The listing builds one solid part. Answer for the finished solid, in the listing's coordinates (mm). Coordinates: 2 decimals unless noted, no trailing zeros. Order: outer loops, then holes, each group sorted by start corner. A loop starts at its lowest first (then second) coordinate and runs counter-clockwise, first axis right, second up. Notation, with made-up numbers: (33.25, -23) -> (47.25, -23) arc R33 ccw to (47.25, 12) -> close; hole circle Ø5 at (-32.75, -23). An arc over 180 degrees is marked (long way). Answer in a Markdown table with one row per item.
```python
from build123d import *

# Parameters (mm, degrees)
F0_W     = 151
F0_H     = 108
F0_R     = 6.5
F0_R_2   = 4.5
F0_R_3   = 3.5
F0_R_4   = 10.35
F0_W_2   = 22
F0_H_2   = 31
F1_DEPTH = 2


with BuildPart() as f1:
    # F0 (on Top) → F1 (new body)
    with BuildSketch(Plane.XY):
        with BuildLine():
            ThreePointArc((50.203704, -19.331837), (45.47278, -13.077209), (38.166667, -15.927249))
            ThreePointArc((38.166667, -15.927249), (41.934628, -25.586465), (50.203704, -19.331837))
        make_face()
        with BuildLine():
            ThreePointArc((50.203704, 39.331837), (41.934628, 45.586465), (38.166667, 35.927249))
            ThreePointArc((38.166667, 35.927249), (45.47278, 33.077209), (50.203704, 39.331837))
        make_face()
        Rectangle(F0_W, F0_H)
        with Locations((-43.3599, -11.497885)):
            Circle(F0_R, mode=Mode.SUBTRACT)
        with Locations((-10, -12.5)):
            Circle(F0_R_2, mode=Mode.SUBTRACT)
        with Locations((10, -27.5)):
            Circle(F0_R_2, mode=Mode.SUBTRACT)
        with BuildLine():
            ThreePointArc((32.203704, -12.260769), (21.611111, -12.941687), (24.5, -2.727922))
            ThreePointArc((24.5, -2.727922), (30.419443, -3.548953), (33.166667, -8.856181))
            ThreePointArc((33.166667, -8.856181), (32.921295, -10.625257), (32.203704, -12.260769))
        make_face(mode=Mode.SUBTRACT)
        with BuildLine():
            ThreePointArc((50.203704, -19.331837), (41.934628, -25.586465), (38.166667, -15.927249))
            ThreePointArc((38.166667, -15.927249), (45.47278, -13.077209), (50.203704, -19.331837))
        make_face(mode=Mode.SUBTRACT)
        with Locations((-50, 10)):
            Circle(F0_R_3, mode=Mode.SUBTRACT)
        with Locations((-29.722222, 0.25004)):
            Circle(F0_R, mode=Mode.SUBTRACT)
        with Locations((-29.722222, 19.74996)):
            Circle(F0_R, mode=Mode.SUBTRACT)
        with Locations((-43.3599, 31.497885)):
            Circle(F0_R, mode=Mode.SUBTRACT)
        with Locations((-62, 42)):
            Circle(F0_R_2, mode=Mode.SUBTRACT)
        with Locations((-5.846048, 33.255358)):
            Circle(F0_R_4, mode=Mode.SUBTRACT)
        with BuildLine():
            ThreePointArc((22.166667, 16.128259), (25.307228, 13.752777), (26.5, 10))
            ThreePointArc((26.5, 10), (25.307228, 6.247223), (22.166667, 3.871741))
            ThreePointArc((22.166667, 3.871741), (13.5, 10), (22.166667, 16.128259))
        make_face(mode=Mode.SUBTRACT)
        with Locations((50, 10)):
            Rectangle(F0_W_2, F0_H_2, mode=Mode.SUBTRACT)
        with BuildLine():
            ThreePointArc((33.166667, 28.856181), (30.419443, 23.548953), (24.5, 22.727922))
            ThreePointArc((24.5, 22.727922), (21.611111, 32.941687), (32.203704, 32.260769))
            ThreePointArc((32.203704, 32.260769), (32.921295, 30.625257), (33.166667, 28.856181))
        make_face(mode=Mode.SUBTRACT)
        with BuildLine():
            ThreePointArc((50.203704, 39.331837), (45.47278, 33.077209), (38.166667, 35.927249))
            ThreePointArc((38.166667, 35.927249), (41.934628, 45.586465), (50.203704, 39.331837))
        make_face(mode=Mode.SUBTRACT)
        with Locations((62, 42)):
            Circle(F0_R_2, mode=Mode.SUBTRACT)
    extrude(amount=F1_DEPTH)


solid = f1.part
```
(1) A flat-ended cylindrical pin translates along its axis: pin 1 (8 mm diameter, centred on x = 20, y = 10, fed in from -Z). Find the tip coordinate at first contact, or state that the pin passes through.
Check values:
| item | result |
|---|---|
| pin 1 | through |
(2) Find the intervals of material crossed by line 1 along Y through (x, z) = (45.5, 0.6); line 2 along Y through (x, z) = (23.5, 1.15); line 3 along X through (y, z) = (2, 0.9), in increasing order. Write a range as from..to.
Check values:
| item | result |
|---|---|
| line 1 | -54..-25.58, -13.08..-5.5, 25.5..33.08, 45.58..54 |
| line 2 | -54..-14.53, -3.18..4.52, 15.48..23.18, 34.53..54 |
| line 3 | -75.5..-35.98, -23.46..39, 61..75.5 |
(3) A cutting plane is placed at B-B, the plane x = -62. Determine the outline of the cut face in (y, z).
Check values:
| item | result |
|---|---|
| outline | (-54, 0) -> (37.5, 0) -> (37.5, 2) -> (-54, 2) -> close; (46.5, 0) -> (54, 0) -> (54, 2) -> (46.5, 2) -> close |
(4) A cutting plane is placed at A-A, the plane y = 42. Determine the outline of the cut face in (x, z).
Check values:
| item | result |
|---|---|
| outline | (-75.5, 0) -> (-66.5, 0) -> (-66.5, 2) -> (-75.5, 2) -> close; (-57.5, 0) -> (-11.38, 0) -> (-11.38, 2) -> (-57.5, 2) -> close; (-0.31, 0) -> (37.78, 0) -> (37.78, 2) -> (-0.31, 2) -> close; (49.63, 0) -> (57.5, 0) -> (57.5, 2) -> (49.63, 2) -> close; (66.5, 0) -> (75.5, 0) -> (75.5, 2) -> (66.5, 2) -> close |
(5) A cutting plane is placed at D-D, the plane x = -8. Determine the outline of the cut face in (y, z).
Check values:
| item | result |
|---|---|
| outline | (-54, 0) -> (-16.53, 0) -> (-16.53, 2) -> (-54, 2) -> close; (-8.47, 0) -> (23.13, 0) -> (23.13, 2) -> (-8.47, 2) -> close; (43.38, 0) -> (54, 0) -> (54, 2) -> (43.38, 2) -> close |
(6) For a pull along X with two mould halves and no side action, classify faces 1 (the cylindrical face through (-48.518, 27.543, 0.986)), 2 (the cylindrical face through (-8.09, 23.15, 0.99)), 3 (the flat face through (-1, 1, 0)) as released by +X, released by -X, zero draft, split by the parting line, or undercut.
Check values:
| item | result |
|---|---|
| face 1 | undercut |
| face 2 | undercut |
| face 3 | zero draft |
(7) A cutting plane is placed at C-C, the plane z = 0.6. Count the separate pieces of the cut face and the enclosed holes in it, then the cut area to 3 significant figures.
Check values:
| item | result |
|---|---|
| separate pieces | 1 |
| enclosed holes | 16 |
| area | 13,800 mm² |
